```python
from build123d import *

# Parameters (mm, degrees)
ESQUISSE1_R             = 5
BOSS_EXTRU_1_DEPTH      = 5
ESQUISSE2_R             = 1.5
BOSS_EXTRU_2_DEPTH      = 2
ESQUISSE3_R             = 1
ENL_V_MAT_EXTRU_1_DEPTH = 10.949874371
ESQUISSE4_R             = 4
ESQUISSE4_R_2           = 3
ENL_V_MAT_EXTRU_2_DEPTH = 2
CONG_1_R                = 1
CONG_2_R                = 1
CONG_3_R                = 0.1


with BuildPart() as part:
    # Esquisse1 → Boss.-Extru.1 (new body)
    with BuildSketch(Plane.XY):
        Circle(ESQUISSE1_R)
    extrude(amount=BOSS_EXTRU_1_DEPTH)

    # Esquisse2 → Boss.-Extru.2 (add)
    with BuildSketch(Plane.XY.offset(5)):
        Circle(ESQUISSE2_R)
    extrude(amount=BOSS_EXTRU_2_DEPTH)

    # Esquisse3 → Enlèv. mat.-Extru.1 (cut, through all)
    with BuildSketch(Plane.XY.offset(7)):
        Circle(ESQUISSE3_R)
    extrude(amount=-ENL_V_MAT_EXTRU_1_DEPTH, mode=Mode.SUBTRACT)

    # Esquisse4 → Enlèv. mat.-Extru.2 (cut)
    with BuildSketch(Plane(origin=(0, 0, 0), x_dir=(-1, 0, 0), z_dir=(0, 0, -1))):
        Circle(ESQUISSE4_R)
        Circle(ESQUISSE4_R_2, mode=Mode.SUBTRACT)
    extrude(amount=-ENL_V_MAT_EXTRU_2_DEPTH, mode=Mode.SUBTRACT)

    # Congé1
    cong_1_edges = [part.edges().sort_by_distance(p)[0] for p in [
        (3, 0, 0),
        (-5, 0, 0),
    ]]
    fillet(cong_1_edges, radius=CONG_1_R - 0.0001)  # a hair under: the kernel refuses the full size

    # Congé2
    cong_2_edges = [part.edges().sort_by_distance(p)[0] for p in [
        (-5, 0, 5),
    ]]
    fillet(cong_2_edges, radius=CONG_2_R)

    # Congé3
    cong_3_edges = [part.edges().sort_by_distance(p)[0] for p in [
        (-1.5, 0, 5),
        (-1.5, 0, 7),
    ]]
    fillet(cong_3_edges, radius=CONG_3_R)


solid = part.part
```
Source: CAD feature listing. Evaluate the final solid. Frame: model axes, mm. A direction names the side the tool comes from. Give positions to 0.01 mm unless a question says otherwise; leave off trailing zeros. Loops run counter-clockwise (first coordinate to the right, second up) from the corner with the lowest first, then second, coordinate; pieces in that order, holes last. Notation, with made-up numbers: (3.5, 44.25) -> (15.5, 44.25) arc R27 ccw to (15.5, 62.25) -> close; hole circle Ø4 at (7, 53). An arc over 180 degrees is marked (long way). Use a Markdown table: item, result. Add a question column.
(1) Pull-direction query (Y, two-part tool) for faces 4 (the face through (0, -1, 4)), 5 (the face through (-1.08, -4.88, 2.48)), 6 (the face through (3, 0.1, 1.5)), 7 (the face through (2, 0, 5)); classes: +Y half, -Y half, draft (parallel to the pull), parting line (faces both ways), or undercut.
(2) Ray query, line 1 (Y direction, x = 0, z = 1.5); line 2 (Y direction, x = 0, z = 5.5); line 3 (Y direction, x = 0, z = 2.75). Return the intervals inside material, ascending.
(3) Section query D-D (z = 3). Output: boundary loops of the cut face in (x, y), then the cut area to 3 significant figures.
(4) First-contact query: pin 1 Ø1 at (x, z) = (3, 5) entering from +Y; pin 2 Ø5 at (x, y) = (3.5, 2.5) entering from +Z. Flat tips, straight axial feed; report the tip coordinate or a pass-through.
(5) Access query for faces 1 (the face through (-1, 3, 2)), 2 (the face through (1, -1, 0)), 3 (the face through (-1.5, 0.07, 5.99)). Directions: +Z, -Z, +X, -X, +Y, -Y. A direction counts if a zero-diameter tool reaches every point of the face in a straight line with its end or side. Return the directions, or none.
(6) Section query C-C (z = 1.5). Output: boundary loops of the cut face in (x, y), then the cut area to 3 significant figures.
Checked values:
| question | item | result |
|---|---|---|
| 1 | face 4 | undercut |
| 1 | face 5 | parting line |
| 1 | face 6 | undercut |
| 1 | face 7 | draft |
| 2 | line 1 | -5 to -4, -3 to -1, 1 to 3, 4 to 5 |
| 2 | line 2 | -1.5 to -1, 1 to 1.5 |
| 2 | line 3 | -5 to -1, 1 to 5 |
| 3 | outline | circle Ø10 at (0, 0); hole circle Ø2 at (0, 0) |
| 3 | area | 75.4 mm^2 |
| 4 | pin 1 | y = 3.97 |
| 4 | pin 2 | z = 5 |
| 5 | face 1 | -Z |
| 5 | face 2 | -Z, +X, -X, +Y, -Y |
| 5 | face 3 | +Z |
| 6 | outline | circle Ø10 at (0, 0); circle Ø6 at (0, 0); hole circle Ø8 at (0, 0); hole circle Ø2 at (0, 0) |
| 6 | area | 53.4 mm^2 |
